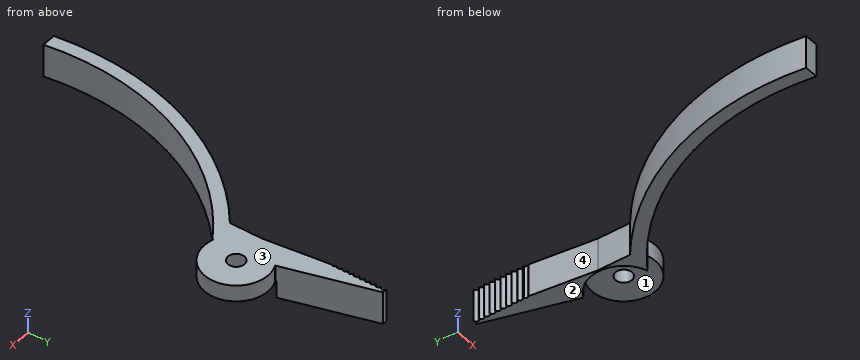
from build123d import *

# Parameters (mm, degrees)
F0_R     = 1.905
F1_DEPTH = 3.81
F2_DEPTH = 3.81
F4_DEPTH = 7.621


# Not quite as in the source:
# - a feature names something its author has since deleted; it is built from what else it names


with BuildPart() as f1:
    # F0 (on Top) → F1 (new body)
    with BuildSketch(Plane.XY):
        with BuildLine():
            ThreePointArc((-28.4269883335, -66.4172298291), (-24.0943230698, -32.9852682882), (-2.3028327904, -7.2637016141))
            Line((-2.3028327904, -7.2637016141), (-7.943934761, -7.4889131964))
            ThreePointArc((-7.943934761, -7.4889131964), (-27.6668151141, -33.7839124183), (-31.6019883335, -66.4172298291))
            Line((-31.6019883335, -66.4172298291), (-28.4269883335, -66.4172298291))
        make_face()
        with BuildLine():
            ThreePointArc((-2.3028327904, -7.2637016141), (-7.6043838567, -0.4875922071), (-3.211656147, 6.9101132258))
            Line((-3.211656147, 6.9101132258), (-10.16, 31.3176262796))
            Line((-10.16, 31.3176262796), (-10.16, 18.6176262796))
            Line((-10.16, 18.6176262796), (-7.943934761, 0))
            Line((-7.943934761, 0), (-7.943934761, -7.4889131964))
            Line((-7.943934761, -7.4889131964), (-2.3028327904, -7.2637016141))
        make_face()
        with BuildLine():
            ThreePointArc((7.366, 0), (3.9446061685, 6.2207747247), (-3.1412055867, 6.6626408775))
            ThreePointArc((-3.1412055867, 6.6626408775), (-7.3521647617, -0.4512530518), (-2.3028327904, -6.9967790546))
            ThreePointArc((-2.3028327904, -6.9967790546), (4.3182918883, -5.9674375713), (7.366, 0))
        make_face()
        Circle(F0_R, mode=Mode.SUBTRACT)
        with BuildLine():
            Line((-3.1412055867, 6.6626408775), (-3.211656147, 6.9101132258))
            ThreePointArc((-3.211656147, 6.9101132258), (-7.6043838567, -0.4875922071), (-2.3028327904, -7.2637016141))
            Line((-2.3028327904, -7.2637016141), (-2.3028327904, -6.9967790546))
            ThreePointArc((-2.3028327904, -6.9967790546), (-7.3521647617, -0.4512530518), (-3.1412055867, 6.6626408775))
        make_face()
    extrude(amount=F1_DEPTH)

    # F0 (on Top) → F2 (join)
    with BuildSketch(Plane.XY):
        with BuildLine():
            ThreePointArc((-2.3028327904, -7.2637016141), (-7.6043838567, -0.4875922071), (-3.211656147, 6.9101132258))
            Line((-3.211656147, 6.9101132258), (-10.16, 31.3176262796))
            Line((-10.16, 31.3176262796), (-10.16, 18.6176262796))
            Line((-10.16, 18.6176262796), (-7.943934761, 0))
            Line((-7.943934761, 0), (-7.943934761, -7.4889131964))
            Line((-7.943934761, -7.4889131964), (-2.3028327904, -7.2637016141))
        make_face()
        with BuildLine():
            ThreePointArc((-28.4269883335, -66.4172298291), (-24.0943230698, -32.9852682882), (-2.3028327904, -7.2637016141))
            Line((-2.3028327904, -7.2637016141), (-7.943934761, -7.4889131964))
            ThreePointArc((-7.943934761, -7.4889131964), (-27.6668151141, -33.7839124183), (-31.6019883335, -66.4172298291))
            Line((-31.6019883335, -66.4172298291), (-28.4269883335, -66.4172298291))
        make_face()
    extrude(amount=-F2_DEPTH)

    # F3 (on face) → F4 (cut, through all)
    with BuildSketch(Plane.XY.offset(3.81)):
        with BuildLine():
            Line((-10.16, 27.284329945), (-10.1133690513, 27.284329945))
            ThreePointArc((-10.1133690513, 27.284329945), (-10.1366687719, 27.2856156574), (-10.16, 27.2860444212))
            Line((-10.16, 27.2860444212), (-10.16, 27.284329945))
        make_face()
        with BuildLine():
            Line((-10.16, 28.5560444212), (-10.16, 27.2860444212))
            ThreePointArc((-10.16, 27.2860444212), (-9.7109871939, 27.4720316151), (-9.525, 27.9210444212))
            ThreePointArc((-9.525, 27.9210444212), (-9.7109871939, 28.3700572272), (-10.16, 28.5560444212))
        make_face()
        with BuildLine():
            Line((-10.1133690513, 27.284329945), (-9.0117990451, 27.284329945))
            Line((-9.0117990451, 27.284329945), (-10.16, 31.3176262796))
            Line((-10.16, 31.3176262796), (-10.16, 28.5560444212))
            ThreePointArc((-10.16, 28.5560444212), (-9.7109871939, 28.3700572272), (-9.525, 27.9210444212))
            ThreePointArc((-9.525, 27.9210444212), (-9.7109871939, 27.4720316151), (-10.16, 27.2860444212))
            ThreePointArc((-10.16, 27.2860444212), (-10.1366687719, 27.2856156574), (-10.1133690513, 27.284329945))
        make_face()
        with BuildLine():
            ThreePointArc((-9.525, 19.0310444212), (-9.7109871939, 19.4800572272), (-10.16, 19.6660444212))
            Line((-10.16, 19.6660444212), (-10.16, 18.6176262796))
            Line((-10.16, 18.6176262796), (-10.1336899082, 18.3965897112))
            ThreePointArc((-10.1336899082, 18.3965897112), (-9.7017795791, 18.5914320398), (-9.525, 19.0310444212))
        make_face()
        with BuildLine():
            Line((-10.16, 27.284329945), (-10.16, 26.0160444212))
            ThreePointArc((-10.16, 26.0160444212), (-9.7109871939, 26.2020316151), (-9.525, 26.6510444212))
            ThreePointArc((-9.525, 26.6510444212), (-9.6947927062, 27.0832563759), (-10.1133690513, 27.284329945))
            Line((-10.1133690513, 27.284329945), (-10.16, 27.284329945))
        make_face()
        with BuildLine():
            Line((-10.16, 26.0160444212), (-10.16, 24.7460444212))
            ThreePointArc((-10.16, 24.7460444212), (-9.7109871939, 24.9320316151), (-9.525, 25.3810444212))
            ThreePointArc((-9.525, 25.3810444212), (-9.7109871939, 25.8300572272), (-10.16, 26.0160444212))
        make_face()
        with BuildLine():
            Line((-10.16, 24.7460444212), (-10.16, 23.4760444212))
            ThreePointArc((-10.1600000026, 23.4760444212), (-9.7109871948, 23.6620316142), (-9.525, 24.1110444212))
            ThreePointArc((-9.525, 24.1110444212), (-9.7109871939, 24.5600572272), (-10.16, 24.7460444212))
        make_face()
        with BuildLine():
            Line((-10.16, 23.4760444212), (-10.16, 22.2060444212))
            ThreePointArc((-10.16, 22.2060444212), (-9.7109871939, 22.3920316151), (-9.525, 22.8410444212))
            ThreePointArc((-9.525, 22.8410444212), (-9.7109871948, 23.2900572282), (-10.1600000026, 23.4760444212))
        make_face()
        with BuildLine():
            Line((-10.16, 22.2060444212), (-10.16, 20.9360444212))
            ThreePointArc((-10.16, 20.9360444212), (-9.7109871939, 21.1220316151), (-9.525, 21.5710444212))
            ThreePointArc((-9.525, 21.5710444212), (-9.7109871939, 22.0200572272), (-10.16, 22.2060444212))
        make_face()
        with BuildLine():
            Line((-10.16, 20.9360444212), (-10.16, 19.6660444212))
            ThreePointArc((-10.16, 19.6660444212), (-9.7109871939, 19.8520316151), (-9.525, 20.3010444212))
            ThreePointArc((-9.525, 20.3010444212), (-9.7109871939, 20.7500572272), (-10.16, 20.9360444212))
        make_face()
        with BuildLine():
            Line((-10.1335594504, 18.3954937079), (-9.9853706378, 17.1505285853))
            ThreePointArc((-9.9853706378, 17.1505285853), (-9.6529917925, 17.3787256046), (-9.525, 17.7610444212))
            ThreePointArc((-9.525, 17.7610444212), (-9.7017343843, 18.20060969), (-10.1335594504, 18.3954937079))
        make_face()
        with BuildLine():
            Line((-9.9793324764, 17.099800732), (-9.8414839109, 15.941706182))
            ThreePointArc((-9.8414839109, 15.941706182), (-9.6097806271, 16.1740528729), (-9.525, 16.4910444212))
            ThreePointArc((-9.525, 16.4910444212), (-9.6511046878, 16.8708477404), (-9.9793324764, 17.099800732))
        make_face()
        with BuildLine():
            ThreePointArc((-9.7032002185, 14.7799560404), (-9.5712331271, 14.9831819202), (-9.525, 15.2210444212))
            ThreePointArc((-9.525, 15.2210444212), (-9.6034746489, 15.5268295313), (-9.8195024679, 15.7570354945))
            Line((-9.8195024679, 15.7570354945), (-9.7032002185, 14.7799560404))
        make_face()
    extrude(amount=-F4_DEPTH, mode=Mode.SUBTRACT)


solid = f1.part
Can you work these out from the model? Positions are in its coordinate system, mm. Face numbers are marked on the shaded views. A direction names the side the tool comes from. Give positions to 0.01 mm unless a question says otherwise; leave off trailing zeros. Write each loop counter-clockwise with the first axis right and the second up, starting at its lowest first coordinate (ties: lowest second). Pieces come first, ordered by that corner, then holes. Notation, with made-up numbers: (58.25, 29) -> (90.25, 29) arc R12 ccw to (90.25, 39) -> close; hole circle Ø3 at (21.5, 53). An arc over 180 degrees is marked (long way). Answer as a JSON object with one key per item and string values. Group by question number.
Item 1: I'm going to push flat-ended pins straight in: P1, Ø6, axis at x = 0, y = 0, coming from the -Z side; P2, Ø1.5, axis at x = -19.5, z = -3, coming from the +Y side; P3, Ø1.5, axis at x = -16, z = -2.5, coming from the -Y side. Where does each tip first touch, or does it pass through?
Item 2: Please list where these lines run through material, in increasing order: line 1 (Y direction, x = 0, z = 2.3) (3 decimals); line 2 (Z direction, x = 4, y = 4); line 3 (X direction, y = -57.5, z = 1.75). Write a range as [from, to].
Item 3: For the marked faces 3 and 4, which set-ups out of +Z, -Z, +X, -X, +Y, -Y let a thin tool reach every point of the face, with its end or its side?
Item 4: Suppose I cut it at D-D (y = -31.5). Please give me the cut outline in (x, z), plus the area to 3 significant figures.
Item 5: We'd pull the mould along Y, two halves only. Please class the marked faces 1 and 2: +Y half, -Y half, draft (parallel to the pull), parting line (faces both ways), or undercut.
Item 6: Suppose I cut it at B-B (x = 0). Please give me the cut outline in (y, z) (3 decimals).
Item 7: Suppose I cut it at C-C (x = -6.5). Please give me the cut outline in (y, z), plus the area to 3 significant figures.
Findings:
{
 "1": {"P1": "stops at z = 0", "P2": "stops at y = -18.31", "P3": "stops at y = -20.64"},
 "2": {"line 1": "y = [-7.366, -1.905], [1.905, 7.366]", "line 2": "z = [0, 3.81]", "line 3": "x = [-32.24, -29.17]"},
 "3": {"face 3": "+Z, +X, -X, +Y, -Y", "face 4": "+Z, -Z, -X"},
 "4": {"outline": "(-26.7, -3.81) -> (-23.41, -3.81) -> (-23.41, 3.81) -> (-26.7, 3.81) -> close", "area": "25.0 mm²"},
 "5": {"face 1": "undercut", "face 2": "draft"},
 "6": {"outline": "(-7.366, 0) -> (-1.905, 0) -> (-1.905, 3.81) -> (-7.366, 3.81) -> close; (1.905, 0) -> (7.366, 0) -> (7.366, 3.81) -> (1.905, 3.81) -> close"},
 "7": {"outline": "(-10.29, -3.81) -> (-3.98, -3.81) -> (-3.98, 0) -> (3.98, 0) -> (3.98, -3.81) -> (18.46, -3.81) -> (18.46, 3.81) -> (-10.29, 3.81) -> close", "area": "189 mm²"}
}
